Input: dimensioned drawing with shaded views. Units: mm. Origin: part minimum x, y, z. Give positions to 0.01 mm unless a question says otherwise; leave off trailing zeros. Loops run counter-clockwise (first coordinate to the right, second up) from the corner with the lowest first, then second, coordinate; pieces in that order, holes last. Notation, with made-up numbers: M 59.5,50 L 95.5,50 A26 cw 95.5,88 Z; hole C 86.5,34 d5. An arc over 180 degrees is marked long. Answer in a Markdown table with one row per item.
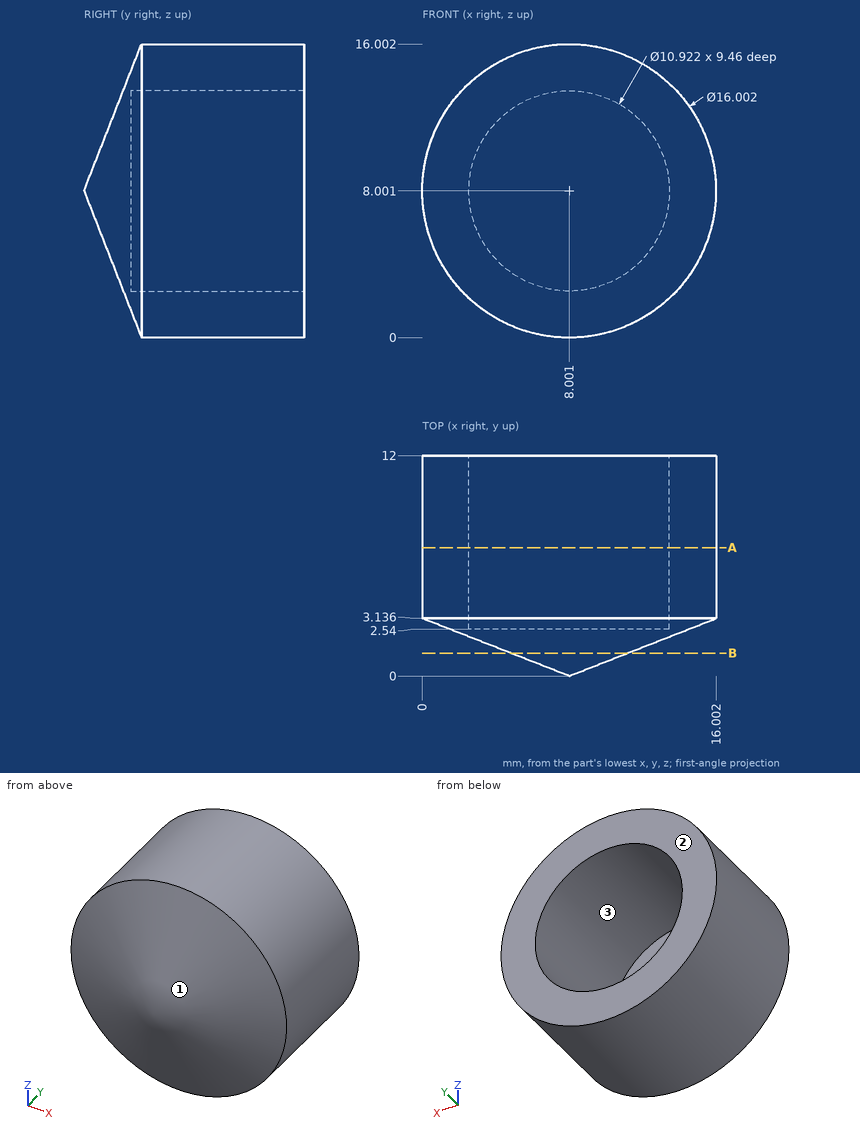
Q1. Section query A-A (y = 7). Output: boundary loops of the cut face in (x, z).
Values follow:
| item | result |
|---|---|
| outline | C 8,8 d16; hole C 8,8 d10.92 |
Q2. Mould query, pull axis Z, two halves, no side actions, for the marked faces 1, 2 and 3. Classes: +Z half, -Z half, draft (parallel to the pull), parting line (faces both ways), or undercut.
Values follow:
| item | result |
|---|---|
| face 1 | parting line |
| face 2 | draft |
| face 3 | undercut |
Q3. Section query B-B (y = 1.25). Output: boundary loops of the cut face in (x, z).
Values follow:
| item | result |
|---|---|
| outline | C 8,8 d6.38 |
Q4. Ray query, probe 1 along X at (y, z) = (10, 9.5); probe 2 along X at (y, z) = (5, 7); probe 3 along Z at (x, y) = (10.5, 5) (1 decimal). Return the intervals inside material, ascending. Write a range as from..to.
Values follow:
| item | result |
|---|---|
| probe 1 | 0.14..2.75, 13.25..15.86 |
| probe 2 | 0.06..2.63, 13.37..15.94 |
| probe 3 | 0.4..3.1, 12.9..15.6 |
Q5. Contact query for flat-ended pins moving along their axis: pin 1 Ø1.5 at (x, y) = (10.5, 5.5) entering from -Z; pin 2 Ø8 at (x, z) = (6.5, 13.5) entering from -Y; pin 3 Ø4 at (x, y) = (11, 6) entering from +Z. Output: stop coordinate, or through.
Values follow:
| item | result |
|---|---|
| pin 1 | z = 0.19 |
| pin 2 | y = 0.67 |
| pin 3 | z = 15.94 |
